Can you work these out from the drawing? Everything is in mm from the part's minimum corner. Give positions to 0.01 mm unless a question says otherwise; leave off trailing zeros. Loops run counter-clockwise (first coordinate to the right, second up) from the corner with the lowest first, then second, coordinate; pieces in that order, holes last. Notation, with made-up numbers: (46.5, 54) - (87.5, 54) arc R25 cw to (87.5, 83) - close; hole circle Ø9 at (1, 78.5). An arc over 180 degrees is marked (long way). One line per item, written item: value. Start each with the question number.
Q1. I want a section at A-A (z = 15). Please give me the cut outline in (x, y).
Q2. I want a section at C-C (y = 1.6). Please give me the cut outline in (x, z), then the cut area to 3 significant figures.
Q3. If I drill on line 1 (Z direction, x = 15, y = 1.25); line 2 (X direction, y = 1.35, z = 7.5), over which ranges is the centre line in solid material (lowest first)? Write a range as from..to.
Q4. I'm going to push a flat-ended pin straight in: P1, Ø1.5, axis at x = 8.5, y = 1.5, coming from the +Z side. Where does the tip first touch, or does it pass through?
Q5. I want a section at B-B (x = 15). Please give me the cut outline in (y, z).
Q6. I want a section at D-D (z = 6.5). Please give me the cut outline in (x, y).
Q7. If we mould it in two halves opening along Z, with no side actions, what happens to the marked faces 1, 2 and 3? For each: released by +Z, released by -Z, zero draft, split by the parting line, or undercut.
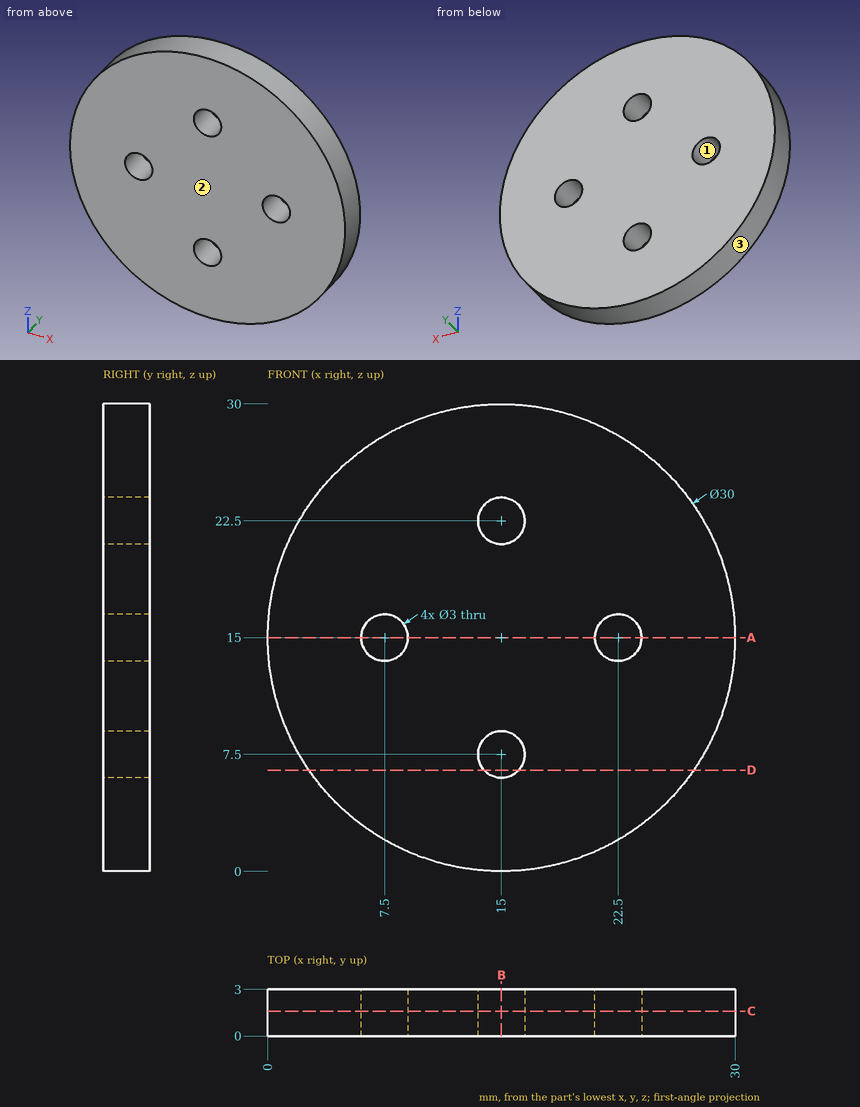
Worked answers:
1. outline: (0, 0) - (6, 0) - (6, 3) - (0, 3) - close; (9, 0) - (21, 0) - (21, 3) - (9, 3) - close; (24, 0) - (30, 0) - (30, 3) - (24, 3) - close
2. outline: circle Ø30 at (15, 15); hole circle Ø3 at (7.5, 15); hole circle Ø3 at (15, 7.5); hole circle Ø3 at (15, 22.5); hole circle Ø3 at (22.5, 15)
2. area: 679 mm²
3. line 1: z = 0..6, 9..21, 24..30
3. line 2: x = 2.01..13.5, 16.5..27.99
4. P1: stops at z = 28.85
5. outline: (0, 0) - (3, 0) - (3, 6) - (0, 6) - close; (0, 9) - (3, 9) - (3, 21) - (0, 21) - close; (0, 24) - (3, 24) - (3, 30) - (0, 30) - close
6. outline: (2.64, 0) - (13.88, 0) - (13.88, 3) - (2.64, 3) - close; (16.12, 0) - (27.36, 0) - (27.36, 3) - (16.12, 3) - close
7. face 1: undercut
7. face 2: zero draft
7. face 3: split by the parting line
